```python
from build123d import *

# Parameters (mm, degrees)
SKETCH1_R           = 1.75
BOSS_EXTRUDE1_DEPTH = 4
SKETCH3_R           = 1.25
CUT_EXTRUDE1_DEPTH  = 38.785297658
CUT_EXTRUDE2_START  = -4
CUT_EXTRUDE2_DEPTH  = 1.5


with BuildPart() as part:
    # Sketch1 → Boss-Extrude1 (new body)
    with BuildSketch(Plane.YZ):
        with BuildLine():
            Line((0.31, 14.63), (-0.31, 14.63))
            ThreePointArc((-0.31, 14.63), (-0.838273314, 13.383704325), (-1.04, 12.04518576))
            ThreePointArc((-1.04, 12.04518576), (-1.578061664, 11.986568374), (-2.112960617, 11.903927815))
            ThreePointArc((-2.112960617, 11.903927815), (-2.65424773, 13.144626757), (-3.487085624, 14.211728743))
            Line((-3.487085624, 14.211728743), (-4.085959636, 14.051260935))
            ThreePointArc((-4.085959636, 14.051260935), (-4.273667417, 12.71070456), (-4.122086336, 11.365584201))
            ThreePointArc((-4.122086336, 11.365584201), (-4.626642697, 11.169703548), (-5.12192646, 10.951436862))
            ThreePointArc((-5.12192646, 10.951436862), (-5.965886177, 12.009764599), (-7.046532125, 12.824951657))
            Line((-7.046532125, 12.824951657), (-7.583467875, 12.514951657))
            ThreePointArc((-7.583467875, 12.514951657), (-7.417818147, 11.171491285), (-6.9232593, 9.911436862))
            ThreePointArc((-6.9232593, 9.911436862), (-7.359925677, 9.591641884), (-7.781841479, 9.252623584))
            ThreePointArc((-7.781841479, 9.252623584), (-8.870959341, 10.05645683), (-10.125769107, 10.564175311))
            Line((-10.125769107, 10.564175311), (-10.564175311, 10.125769107))
            ThreePointArc((-10.564175311, 10.125769107), (-10.05645683, 8.870959341), (-9.252623584, 7.781841479))
            ThreePointArc((-9.252623584, 7.781841479), (-9.591641884, 7.359925677), (-9.911436862, 6.9232593))
            ThreePointArc((-9.911436862, 6.9232593), (-11.171491285, 7.417818147), (-12.514951657, 7.583467875))
            Line((-12.514951657, 7.583467875), (-12.824951657, 7.046532125))
            ThreePointArc((-12.824951657, 7.046532125), (-12.009764599, 5.965886177), (-10.951436862, 5.12192646))
            ThreePointArc((-10.951436862, 5.12192646), (-11.169703548, 4.626642697), (-11.365584201, 4.122086336))
            ThreePointArc((-11.365584201, 4.122086336), (-12.71070456, 4.273667417), (-14.051260935, 4.085959636))
            Line((-14.051260935, 4.085959636), (-14.211728743, 3.487085624))
            ThreePointArc((-14.211728743, 3.487085624), (-13.144626757, 2.65424773), (-11.903927815, 2.112960617))
            ThreePointArc((-11.903927815, 2.112960617), (-11.986568374, 1.578061664), (-12.04518576, 1.04))
            ThreePointArc((-12.04518576, 1.04), (-13.383704325, 0.838273314), (-14.63, 0.31))
            Line((-14.63, 0.31), (-14.63, -0.31))
            ThreePointArc((-14.63, -0.31), (-13.383704325, -0.838273314), (-12.04518576, -1.04))
            ThreePointArc((-12.04518576, -1.04), (-11.986568374, -1.578061664), (-11.903927815, -2.112960617))
            ThreePointArc((-11.903927815, -2.112960617), (-13.144626757, -2.65424773), (-14.211728743, -3.487085624))
            Line((-14.211728743, -3.487085624), (-14.051260935, -4.085959636))
            ThreePointArc((-14.051260935, -4.085959636), (-12.71070456, -4.273667417), (-11.365584201, -4.122086336))
            ThreePointArc((-11.365584201, -4.122086336), (-11.169703548, -4.626642697), (-10.951436862, -5.12192646))
            ThreePointArc((-10.951436862, -5.12192646), (-12.009764599, -5.965886177), (-12.824951657, -7.046532125))
            Line((-12.824951657, -7.046532125), (-12.514951657, -7.583467875))
            ThreePointArc((-12.514951657, -7.583467875), (-11.171491285, -7.417818147), (-9.911436862, -6.9232593))
            ThreePointArc((-9.911436862, -6.9232593), (-9.591641884, -7.359925677), (-9.252623584, -7.781841479))
            ThreePointArc((-9.252623584, -7.781841479), (-10.05645683, -8.870959341), (-10.564175311, -10.125769107))
            Line((-10.564175311, -10.125769107), (-10.125769107, -10.564175311))
            ThreePointArc((-10.125769107, -10.564175311), (-8.870959341, -10.05645683), (-7.781841479, -9.252623584))
            ThreePointArc((-7.781841479, -9.252623584), (3.191677838, -11.661101688), (11.409123542, -4))
            ThreePointArc((11.409123542, -4), (11.561502637, -3.438555035), (11.740713538, -2.885090229))
            Line((11.740713538, -2.885090229), (13.278503475, -2.736624135))
            Line((13.278503475, -2.736624135), (30.992077522, -1.026465229))
            ThreePointArc((30.992077522, -1.026465229), (34.589171795, 3.3394153), (30.223291266, 6.936509573))
            Line((30.223291266, 6.936509573), (10.971927281, 5.077884573))
            ThreePointArc((10.971927281, 5.077884573), (10.96170419, 5.099915807), (10.951436862, 5.12192646))
            ThreePointArc((10.951436862, 5.12192646), (12.009764599, 5.965886177), (12.824951657, 7.046532125))
            Line((12.824951657, 7.046532125), (12.514951657, 7.583467875))
            ThreePointArc((12.514951657, 7.583467875), (11.171491285, 7.417818147), (9.911436862, 6.9232593))
            ThreePointArc((9.911436862, 6.9232593), (9.591641884, 7.359925677), (9.252623584, 7.781841479))
            ThreePointArc((9.252623584, 7.781841479), (10.05645683, 8.870959341), (10.564175311, 10.125769107))
            Line((10.564175311, 10.125769107), (10.125769107, 10.564175311))
            ThreePointArc((10.125769107, 10.564175311), (8.870959341, 10.05645683), (7.781841479, 9.252623584))
            ThreePointArc((7.781841479, 9.252623584), (7.359925677, 9.591641884), (6.9232593, 9.911436862))
            ThreePointArc((6.9232593, 9.911436862), (7.417818147, 11.171491285), (7.583467875, 12.514951657))
            Line((7.583467875, 12.514951657), (7.046532125, 12.824951657))
            ThreePointArc((7.046532125, 12.824951657), (5.965886177, 12.009764599), (5.12192646, 10.951436862))
            ThreePointArc((5.12192646, 10.951436862), (4.626642697, 11.169703548), (4.122086336, 11.365584201))
            ThreePointArc((4.122086336, 11.365584201), (4.273667417, 12.71070456), (4.085959636, 14.051260935))
            Line((4.085959636, 14.051260935), (3.487085624, 14.211728743))
            ThreePointArc((3.487085624, 14.211728743), (2.65424773, 13.144626757), (2.112960617, 11.903927815))
            ThreePointArc((2.112960617, 11.903927815), (1.578061664, 11.986568374), (1.04, 12.04518576))
            ThreePointArc((1.04, 12.04518576), (0.838273314, 13.383704325), (0.31, 14.63))
        make_face()
        with Locations(Location((0, 0, 0), (0, 0, 270))):
            Circle(SKETCH1_R, mode=Mode.SUBTRACT)
        with Locations(Location((30.607684394, 2.955022172, 0), (0, 0, 270))):
            Circle(SKETCH1_R, mode=Mode.SUBTRACT)
    extrude(amount=BOSS_EXTRUDE1_DEPTH)

    # Sketch3 → Cut-Extrude1 (cut, through all)
    with BuildSketch(Plane(origin=(0, 0, 0), x_dir=(0, -1, 0), z_dir=(-1, 0, 0))):
        with Locations(Location((-4.479173326, 0.432442269, 0), (0, 0, 90))):
            Circle(SKETCH3_R)
        with Locations(Location((4.479173326, -0.432442269, 0), (0, 0, 270))):
            Circle(SKETCH3_R)
    extrude(amount=-CUT_EXTRUDE1_DEPTH, mode=Mode.SUBTRACT)

    # Sketch4 → Cut-Extrude2 (cut)
    with BuildSketch(Plane(origin=(0, 0, 0), x_dir=(0, -1, 0), z_dir=(-1, 0, 0)).offset(CUT_EXTRUDE2_START)):
        with BuildLine():
            ThreePointArc((6.229173326, -0.432442269), (5.774704296, 0.744035315), (4.647345319, 1.309458469))
            Line((4.647345319, 1.309458469), (4.311001332, -2.174343007))
            ThreePointArc((4.311001332, -2.174343007), (5.65565091, -1.727973239), (6.229173326, -0.432442269))
        make_face()
        with BuildLine():
            Line((4.311001332, -2.174343007), (4.647345319, 1.309458469))
            ThreePointArc((4.647345319, 1.309458469), (2.737272588, -0.264270276), (4.311001332, -2.174343007))
        make_face()
        with BuildLine():
            ThreePointArc((-2.729173326, 0.432442269), (-3.183642356, 1.608919853), (-4.311001332, 2.174343007))
            Line((-4.311001332, 2.174343007), (-4.647345319, -1.309458469))
            ThreePointArc((-4.647345319, -1.309458469), (-3.302695742, -0.863088701), (-2.729173326, 0.432442269))
        make_face()
        with BuildLine():
            Line((-4.647345319, -1.309458469), (-4.311001332, 2.174343007))
            ThreePointArc((-4.311001332, 2.174343007), (-6.221074064, 0.600614263), (-4.647345319, -1.309458469))
        make_face()
        with BuildLine():
            ThreePointArc((4.311001332, -2.174343007), (2.737272588, -0.264270276), (4.647345319, 1.309458469))
            Line((4.647345319, 1.309458469), (-4.311001332, 2.174343007))
            ThreePointArc((-4.311001332, 2.174343007), (-3.183642356, 1.608919853), (-2.729173326, 0.432442269))
            ThreePointArc((-2.729173326, 0.432442269), (-3.302695742, -0.863088701), (-4.647345319, -1.309458469))
            Line((-4.647345319, -1.309458469), (4.311001332, -2.174343007))
        make_face()
    extrude(amount=CUT_EXTRUDE2_DEPTH, mode=Mode.SUBTRACT)


solid = part.part
```
Can you work these out from the model? Positions are in its coordinate system, mm. A direction names the side the tool comes from. Coordinates: 2 decimals unless noted, no trailing zeros. Loops run counter-clockwise (first coordinate to the right, second up) from the corner with the lowest first, then second, coordinate; pieces in that order, holes last.
Item 1: Suppose I cut it at B-B (y = 27.5). Please give me the cut outline in (x, z), then the cut area to 3 significant figures.
Answers below:
outline: (0, -1.36) - (4, -1.36) - (4, 6.67) - (0, 6.67) - close
area: 32.1 mm2
Item 2: If we mould it in two halves opening along Z, with no side actions, what happens to faces 4 (the face through (0, 4, -2)), 5 (the face through (1.972, -4.273, 12.73)), 6 (the face through (1.972, -1.571, 11.988))? For each: released by +Z, released by -Z, zero draft, split by the parting line, or undercut.
Answers below:
face 4: zero draft
face 5: undercut
face 6: released by +Z
Item 3: I'm going to push flat-ended pins straight in: pin 1 (1 mm diameter, centred on x = 2.5, y = -7.5, fed in from -Z); pin 2 (3 mm diameter, centred on y = -4.48, z = -0.43, fed in from +X). Where does each tip first touch, or does it pass through?
Answers below:
pin 1: stops at z = -9.86
pin 2: stops at x = 2.5
Item 4: Please list where these lines run through material, in increasing order: L1, parallel to Z at x = 0.9, y = 0; L2, parallel to Z at x = 2.9, y = 0; L3, parallel to Y at x = 3.5, z = 12.5.
Answers below:
L1: z = -12.09 to -1.75, 1.75 to 14.63
L2: z = -12.09 to -1.76, 1.76 to 14.63
L3: y = -7.58 to -6.55, -4.27 to -2.33, -1.01 to 1.01, 2.33 to 4.27, 6.55 to 7.58
Item 5: Which directions (+Z, -Z, +X, -X, +Y, -Y) give clear straight access to the entire face, cutting with the end or side of a thin tool? Please do faces 1 (the face through (1.972, 10.047, 8.854)), 2 (the face through (1.972, -12.023, 5.98)), 3 (the face through (1.972, 2.664, 13.161)).
Answers below:
face 1: +X, -X, +Y
face 2: +X, -X, -Y
face 3: +Z, +X, -X
Item 6: Suppose I cut it at A-A (x = 0.9). State how many separate pieces and enclosed holes the cut face has, then the cut area to 3 significant figures.
Answers below:
separate pieces: 1
enclosed holes: 4
area: 663 mm2
